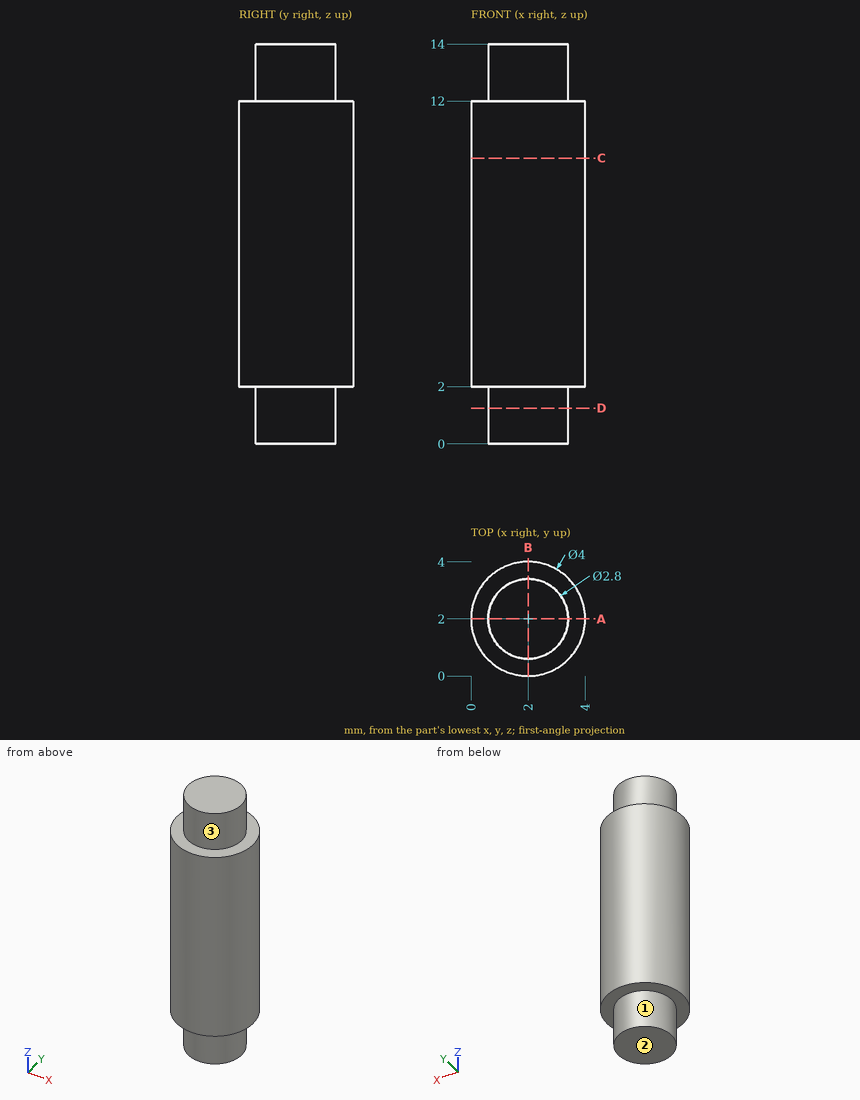
Study the drawing (mm; zero at the part's minimum x, y, z) and answer. A direction names the side the tool comes from. Give positions to 0.01 mm unless a question says otherwise; leave off trailing zeros. Order: outer loops, then holes, each group sorted by start corner. A loop starts at its lowest first (then second) coordinate and runs counter-clockwise, first axis right, second up. Notation, with made-up numbers: (61, 89.25) -> (77, 89.25) arc R14 ccw to (77, 116.25) -> close; hole circle Ø11 at (10.5, 24.25). An arc over 180 degrees is marked (long way). Write item = value, one per line.
1. A cutting plane is placed at C-C, the plane z = 10. Write down the section's boundary in (x, y), and give its area (3 significant figures).
Numbers:
outline = circle Ø4 at (2, 2)
area = 12.6 mm²
2. Straight lines are drawn through the part: line 1 along Z through (x, y) = (3.6, 1.8); line 2 along Y through (x, z) = (2.25, 0.75); line 3 along X through (y, z) = (2, 13.25). For each, find the intervals that lie inside material, in ascending order.
Numbers:
line_1 = 2 to 12
line_2 = 0.62 to 3.38
line_3 = 0.6 to 3.4
3. A cutting plane is placed at A-A, the plane y = 2. Write down the section's boundary in (x, z), and give its area (3 significant figures).
Numbers:
outline = (0, 2) -> (0.6, 2) -> (0.6, 0) -> (3.4, 0) -> (3.4, 2) -> (4, 2) -> (4, 12) -> (3.4, 12) -> (3.4, 14) -> (0.6, 14) -> (0.6, 12) -> (0, 12) -> close
area = 51.2 mm²
4. A cutting plane is placed at D-D, the plane z = 1.25. Write down the section's boundary in (x, y).
Numbers:
outline = circle Ø2.8 at (2, 2)
5. For the marked faces 1, 2 and 3, determine the directions among +Z, -Z, +X, -X, +Y, -Y from which every point of the face is accessible in a straight line to the end or side of a thin tool.
Numbers:
face_1 = -Z
face_2 = -Z, +X, -X, +Y, -Y
face_3 = +Z
